from build123d import *

# Parameters (mm, degrees)
SKETCH1_R          = 9
EXTRUDE1_DEPTH     = 2
SKETCH4_R          = 7
EXTRUDE2_DEPTH     = 19
SKETCH2_R          = 5.5
CUT_EXTRUDE1_DEPTH = 10
SKETCH3_R          = 7.8
SKETCH3_R_2        = 7
CUT_EXTRUDE2_DEPTH = 1
SKETCH5_R          = 5
EXTRUDE3_DEPTH     = 8.5
SKETCH6_R          = 0.35
CUT_EXTRUDE3_DEPTH = 7
CHAMFER2_SIZE      = 0.15
CHAMFER1_SIZE      = 0.2
SKETCH7_R          = 5
CUT_EXTRUDE4_DEPTH = 1
CHAMFER3_SIZE      = 0.5
EXTRUDE4_DEPTH     = 3


with BuildPart() as part:
    # Sketch1 → Extrude1 (new body)
    with BuildSketch(Plane.XY):
        Circle(SKETCH1_R)
    extrude(amount=EXTRUDE1_DEPTH)

    # Sketch4 → Extrude2 (add)
    with BuildSketch(Plane(origin=(0, 0, 0), x_dir=(-1, 0, 0), z_dir=(0, 0, -1))):
        Circle(SKETCH4_R)
    extrude(amount=EXTRUDE2_DEPTH)

    # Sketch2 → Cut-Extrude1 (cut)
    with BuildSketch(Plane.XY.offset(2)):
        Circle(SKETCH2_R)
    extrude(amount=-CUT_EXTRUDE1_DEPTH, mode=Mode.SUBTRACT)

    # Sketch3 → Cut-Extrude2 (cut)
    with BuildSketch(Plane(origin=(0, 0, 0), x_dir=(-1, 0, 0), z_dir=(0, 0, -1))):
        Circle(SKETCH3_R)
        Circle(SKETCH3_R_2, mode=Mode.SUBTRACT)
    extrude(amount=-CUT_EXTRUDE2_DEPTH, mode=Mode.SUBTRACT)

    # Sketch5 → Extrude3 (add)
    with BuildSketch(Plane.XY.offset(-8)):
        Circle(SKETCH5_R)
    extrude(amount=EXTRUDE3_DEPTH)

    # Sketch6 → Cut-Extrude3 (cut)
    with BuildSketch(Plane.XY.offset(0.5)):
        with Locations((0, 3)):
            Circle(SKETCH6_R)
        with Locations((0, -3)):
            Circle(SKETCH6_R)
        with Locations((2.121320344, 2.121320344)):
            Circle(SKETCH6_R)
        with Locations((2.121320344, -2.121320344)):
            Circle(SKETCH6_R)
        with Locations((-2.121320344, 2.121320344)):
            Circle(SKETCH6_R)
        with Locations((-2.121320344, -2.121320344)):
            Circle(SKETCH6_R)
        with Locations((-3, 0)):
            Circle(SKETCH6_R)
        with Locations((3, 0)):
            Circle(SKETCH6_R)
    extrude(amount=-CUT_EXTRUDE3_DEPTH, mode=Mode.SUBTRACT)

    # Chamfer2
    chamfer2_edges = [part.edges().sort_by_distance(p)[0] for p in [
        (-5, 0, 0.5),
        (-0.35, 3, 0.5),
        (-0.35, -3, 0.5),
        (1.771320344, 2.121320344, 0.5),
        (1.771320344, -2.121320344, 0.5),
        (-2.471320344, 2.121320344, 0.5),
        (-2.471320344, -2.121320344, 0.5),
        (-3.35, 0, 0.5),
        (2.65, 0, 0.5),
    ]]
    chamfer(chamfer2_edges, length=CHAMFER2_SIZE)

    # Chamfer1
    chamfer1_edges = [part.edges().sort_by_distance(p)[0] for p in [
        (-5.5, 0, 2),
        (-9, 0, 2),
    ]]
    chamfer(chamfer1_edges, length=CHAMFER1_SIZE)

    # Sketch7 → Cut-Extrude4 (cut)
    with BuildSketch(Plane(origin=(0, 0, -19), x_dir=(-1, 0, 0), z_dir=(0, 0, -1))):
        Circle(SKETCH7_R)
    extrude(amount=-CUT_EXTRUDE4_DEPTH, mode=Mode.SUBTRACT)

    # Chamfer3
    chamfer3_edges = [part.edges().sort_by_distance(p)[0] for p in [
        (7, 0, -19),
    ]]
    chamfer(chamfer3_edges, length=CHAMFER3_SIZE)

    # Sketch9 → Extrude4 (add)
    with BuildSketch(Plane(origin=(0, 0, -18), x_dir=(-1, 0, 0), z_dir=(0, 0, -1))):
        Polygon((-4.907477288, 8.5), (4.907477288, 8.5), (9.814954576, 0), (4.907477288, -8.5), (-4.907477288, -8.5), (-9.814954576, 0), align=None)
    extrude(amount=-EXTRUDE4_DEPTH)


solid = part.part
Here's how the part is built. I have some questions about the finished solid (model axes, mm). A direction names the side the tool comes from. Round coordinates to 2 decimals unless told otherwise and drop trailing zeros. Write each loop counter-clockwise with the first axis right and the second up, starting at its lowest first coordinate (ties: lowest second). Pieces come first, ordered by that corner, then holes. Notation, with made-up numbers: (-24, -20.5) -> (1, -20.5) arc R21 ccw to (1, 13.5) -> close; hole circle Ø6 at (82.5, -18.75). An arc over 180 degrees is marked (long way). One line per item, written item: value.
1) I'm going to push flat-ended pins straight in: pin 1 Ø0.6 at (x, y) = (-2, -2) entering from +Z; pin 2 Ø6 at (x, z) = (1.5, -11.5) entering from -Y; pin 3 Ø9 at (x, y) = (0.5, 1) entering from +Z; pin 4 Ø9 at (x, y) = (2, 1) entering from -Z. Where does each tip first touch, or does it pass through?
Filled sheet:
pin 1: stops at z = 0.47
pin 2: stops at y = -7
pin 3: stops at z = 1.92
pin 4: stops at z = -19
2) For faces 4 (the face through (-7.327, 4.309, -16.521)), 5 (the face through (-7, 4, 0)), 6 (the face through (0, -8.5, -17)), which set-ups out of +Z, -Z, +X, -X, +Y, -Y let a thin tool reach every point of the face, with its end or its side?
Filled sheet:
face 4: -Z, -X, +Y
face 5: none
face 6: -Z, +X, -X, -Y
3) Suppose I cut it at B-B on z = -7. List the corners of the cut face in (x, y) for me.
Filled sheet:
outline: circle Ø14 at (0, 0); circle Ø10 at (0, 0); hole circle Ø11 at (0, 0)
4) If I drill on line 1 (Y direction, x = 4, z = -1.5); line 2 (Z direction, x = -6.25, y = 6); line 3 (Y direction, x = 0, z = -18.2), over which ranges is the centre line in solid material (lowest first)? Write a range as [from, to].
Filled sheet:
line 1: y = [-5.74, -3.77], [-3, 3], [3.77, 5.74]
line 2: z = [-18, -15], [0, 2]
line 3: y = [-7, -5], [5, 7]
5) Suppose I cut it at C-C on z = -11. List the corners of the cut face in (x, y) for me, plus the area to 3 significant figures.
Filled sheet:
outline: circle Ø14 at (0, 0)
area: 154 mm2
6) We'd pull the mould along X, two halves only. Please class faces 1 (the face through (1.08, -4.88, -18.51)), 2 (the face through (7.327, -4.309, -16.521)), 3 (the face through (0, 8.5, -17)): released by +X, released by -X, zero draft, split by the parting line, or undercut.
Filled sheet:
face 1: undercut
face 2: released by +X
face 3: zero draft
7) Suppose I cut it at A-A on z = -3.5. Give the number of separate pieces and of enclosed holes in the cut face, plus the area to 3 significant figures.
Filled sheet:
separate pieces: 2
enclosed holes: 9
area: 134 mm2
